```python
from build123d import *

# Parameters (mm, degrees)
F0_W     = 94.654716
F0_H     = 113.359868
F1_DEPTH = 25.4
F2_R     = 29.109761
F3_DEPTH = 25.401
F4_R     = 5.08
F5_R     = 10


with BuildPart() as f1:
    # F0 (on Top) → F1 (new body)
    with BuildSketch(Plane.XY):
        Rectangle(F0_W, F0_H)
    extrude(amount=F1_DEPTH)

    # F2 (on face) → F3 (cut, through all)
    with BuildSketch(Plane.XY.offset(25.4)):
        Circle(F2_R)
    extrude(amount=-F3_DEPTH, mode=Mode.SUBTRACT)

    # F4
    f4_edges = [f1.edges().sort_by_distance(p)[0] for p in [
        (-47.327358, -56.679934, 12.7),
        (47.327358, -56.679934, 12.7),
        (0, -56.679934, 0),
        (0, -56.679934, 25.4),
        (47.327358, 56.679934, 12.7),
        (47.327358, 0, 0),
        (47.327358, 0, 25.4),
        (-47.327358, 56.679934, 12.7),
        (0, 56.679934, 0),
        (0, 56.679934, 25.4),
        (-47.327358, 0, 0),
        (-47.327358, 0, 25.4),
    ]]
    fillet(f4_edges, radius=F4_R)

    # F5
    f5_edges = [f1.edges().sort_by_distance(p)[0] for p in [
        (-29.109761, 0, 25.4),
        (29.109761, 0, 12.7),
        (-29.109761, 0, 0),
    ]]
    fillet(f5_edges, radius=F5_R)


solid = f1.part
```
The listing builds one solid part. Answer for the finished solid, in the listing's coordinates (mm). Coordinates: 2 decimals unless noted, no trailing zeros. Write each loop counter-clockwise with the first axis right and the second up, starting at its lowest first coordinate (ties: lowest second). Pieces come first, ordered by that corner, then holes. Notation, with made-up numbers: (86, 86.5) - (90, 86.5) arc R11 cw to (90, 99.5) - close; hole circle Ø5 at (87, -0.5). An arc over 180 degrees is marked (long way). Return JSON: item names as keys, results as strings. Group by question number.
Q1. The part is cut by section B-B on z = 12. Write down the section's boundary in (x, y), and give its area (3 significant figures).
Q2. For a pull along X with two mould halves and no side action, classify faces 1 (the cylindrical face through (45.8, 0.72, 1.45)), 2 (the flat face through (-19, 35, 25.4)), 3 (the cylindrical face through (27.766, 8.744, 12.738)) as +X half, -X half, draft (parallel to the pull), parting line (faces both ways), or undercut.
Q3. A flat-ended cylindrical pin translates along its axis: pin 1 Ø6 at (x, y) = (-14, 30.5) entering from +Z. Find the tip coordinate at first contact, or state that the pin passes through.
Q4. The part is cut by section C-C on y = 0. Write down the section's boundary in (x, z).
Q5. Find the intervals of material crossed by line 1 along Y through (x, z) = (0, 11.55); line 2 along Y through (x, z) = (-18, 15.5); line 3 along Y through (x, z) = (35, 5), in increasing order. Write a range as [from, to].
Q6. The part is cut by section A-A on x = 0. Write down the section's boundary in (y, z).
Evaluation:
{
 "1": {"outline": "(-47.33, -51.6) arc R5.08 ccw to (-42.25, -56.68) - (42.25, -56.68) arc R5.08 ccw to (47.33, -51.6) - (47.33, 51.6) arc R5.08 ccw to (42.25, 56.68) - (-42.25, 56.68) arc R5.08 ccw to (-47.33, 51.6) - close; hole circle Ø58.22 at (0, 0)", "area": "8,050 mm2"},
 "2": {"face 1": "+X half", "face 2": "draft", "face 3": "undercut"},
 "3": {"pin 1": "stops at z = 25.07"},
 "4": {"outline": "(-47.33, 5.08) arc R5.08 ccw to (-42.25, 0) - (-39.11, 0) arc R10 ccw to (-29.11, 10) - (-29.11, 15.4) arc R10 ccw to (-39.11, 25.4) - (-42.25, 25.4) arc R5.08 ccw to (-47.33, 20.32) - close; (29.11, 10) arc R10 ccw to (39.11, 0) - (42.25, 0) arc R5.08 ccw to (47.33, 5.08) - (47.33, 20.32) arc R5.08 ccw to (42.25, 25.4) - (39.11, 25.4) arc R10 ccw to (29.11, 15.4) - close"},
 "5": {"line 1": "y = [-56.68, -29.11], [29.11, 56.68]", "line 2": "y = [-56.68, -22.88], [22.88, 56.68]", "line 3": "y = [-56.68, 56.68]"},
 "6": {"outline": "(-56.68, 5.08) arc R5.08 ccw to (-51.6, 0) - (-39.11, 0) arc R10 ccw to (-29.11, 10) - (-29.11, 15.4) arc R10 ccw to (-39.11, 25.4) - (-51.6, 25.4) arc R5.08 ccw to (-56.68, 20.32) - close; (29.11, 10) arc R10 ccw to (39.11, 0) - (51.6, 0) arc R5.08 ccw to (56.68, 5.08) - (56.68, 20.32) arc R5.08 ccw to (51.6, 25.4) - (39.11, 25.4) arc R10 ccw to (29.11, 15.4) - close"}
}
